Part model, mm, in its own coordinate system. A direction names the side the tool comes from. Give positions to 0.01 mm unless a question says otherwise; leave off trailing zeros. Write each loop counter-clockwise with the first axis right and the second up, starting at its lowest first coordinate (ties: lowest second). Pieces come first, ordered by that corner, then holes. Notation, with made-up numbers: M 85,8.25 L 99,8.25 A9 cw 99,20.25 Z; hole C 66.5,8 d3. An arc over 180 degrees is marked long. Use a Markdown table: item, result. Add a question column.
from build123d import *

# Parameters (mm, degrees)
SKETCH1_W            = 33
SKETCH1_H            = 29
BOSS_EXTRUDE1_DEPTH  = 2
SKETCH2_W            = 33
SKETCH2_H            = 29
SKETCH2_W_2          = 29
SKETCH2_H_2          = 25
BOSS_EXTRUDE2_DEPTH  = 10.5
SKETCH4_W            = 7.5
SKETCH4_H            = 6
CUT_EXTRUDE1_DEPTH   = 2
FILLET1_R            = 2
SKETCH5_W            = 8
SKETCH5_H            = 1
CUT_EXTRUDE2_DEPTH   = 31
FILLET2_R            = 0.5
FILLET2_OF_MIRROR1_R = 0.5


with BuildPart() as part:
    # Sketch1 → Boss-Extrude1 (new body)
    with BuildSketch(Plane(origin=(0, 0, 0), x_dir=(1, 0, 0), z_dir=(0, 1, 0))):
        Rectangle(SKETCH1_W, SKETCH1_H)
    extrude(amount=BOSS_EXTRUDE1_DEPTH)

    # Sketch2 → Boss-Extrude2 (add)
    with BuildSketch(Plane(origin=(0, 2, 0), x_dir=(1, 0, 0), z_dir=(0, 1, 0))):
        Rectangle(SKETCH2_W, SKETCH2_H)
        Rectangle(SKETCH2_W_2, SKETCH2_H_2, mode=Mode.SUBTRACT)
    extrude(amount=BOSS_EXTRUDE2_DEPTH)

    # Sketch4 → Cut-Extrude1 (cut)
    with BuildSketch(Plane(origin=(0, 2, 0), x_dir=(1, 0, 0), z_dir=(0, 1, 0))):
        with Locations((0.05, 4.5)):
            Rectangle(SKETCH4_W, SKETCH4_H)
    extrude(amount=-CUT_EXTRUDE1_DEPTH, mode=Mode.SUBTRACT)

    # Fillet1
    fillet1_edges = [part.edges().sort_by_distance(p)[0] for p in [
        (14.5, 7.25, -12.5),
        (-14.5, 7.25, -12.5),
        (-14.5, 7.25, 12.5),
        (14.5, 7.25, 12.5),
        (16.5, 6.25, 14.5),
        (-16.5, 6.25, 14.5),
        (-16.5, 6.25, -14.5),
        (16.5, 6.25, -14.5),
    ]]
    fillet(fillet1_edges, radius=FILLET1_R)

    # Sketch5 → Cut-Extrude2 (cut)
    with BuildSketch(Plane(origin=(16.5, 0, 0), x_dir=(0, 0, -1), z_dir=(1, 0, 0))):
        with Locations((0, 12)):
            Rectangle(SKETCH5_W, SKETCH5_H)
    cut_extrude2 = extrude(amount=-CUT_EXTRUDE2_DEPTH, mode=Mode.SUBTRACT)

    # Fillet2
    fillet2_edges = [part.edges().sort_by_distance(p)[0] for p in [
        (15.5, 11.5, 4),
        (15.5, 11.5, -4),
    ]]
    fillet(fillet2_edges, radius=FILLET2_R)

    # Mirror1: Cut-Extrude2 across plane
    add(cut_extrude2.mirror(Plane(origin=(0, 0, 0), x_dir=(0, 0, 1), z_dir=(1, 0, 0))), mode=Mode.SUBTRACT)

    # Fillet2 of Mirror1
    fillet2_of_mirror1_edges = [part.edges().sort_by_distance(p)[0] for p in [
        (-15.5, 11.5, 4),
        (-15.5, 11.5, -4),
    ]]
    fillet(fillet2_of_mirror1_edges, radius=FILLET2_OF_MIRROR1_R)


solid = part.part
1. Cut at A-A (x = -1.5). Write the cut outline in (y, z), then the cut area to 3 significant figures.
2. Cut at C-C (y = 3.5). Write the cut outline in (x, z).
3. Tool access for faces 1 (the flat face through (0, 7, 12.5)), 2 (the flat face through (0, 1, -7.5)), 3 (the flat face through (-16, 11.5, 0)): list every direction of +Z, -Z, +X, -X, +Y, -Y with a clear straight run to the whole face (end or side of a thin tool).
4. Drill centre lines: probe 1 along X at (y, z) = (4.75, -9.25); probe 2 along Z at (x, y) = (3, 7); probe 3 along X at (y, z) = (1.5, -2). Where is each one in solid material? Low to high. Write a range as [from, to].
5. Flat gauge pins, fed straight in: pin 1 (1 mm diameter, centred on x = 15.5, z = 1, fed in from +Y); pin 2 (3 mm diameter, centred on x = -10, z = 0, fed in from +Y). Where does each tip first touch, or does it go through?
6. Cut at B-B (z = 8.5). Write the cut outline in (x, y).
7. Cut at D-D (z = -6.25). Write the cut outline in (x, y).
A:
| question | item | result |
|---|---|---|
| 1 | outline | M 0,-14.5 L 12.5,-14.5 L 12.5,-12.5 L 2,-12.5 L 2,-7.5 L 0,-7.5 Z; M 0,-1.5 L 2,-1.5 L 2,12.5 L 12.5,12.5 L 12.5,14.5 L 0,14.5 Z |
| 1 | area | 88.0 mm² |
| 2 | outline | M -16.5,-12.5 A2 ccw -14.5,-14.5 L 14.5,-14.5 A2 ccw 16.5,-12.5 L 16.5,12.5 A2 ccw 14.5,14.5 L -14.5,14.5 A2 ccw -16.5,12.5 Z; hole M -14.5,-10.5 A2 ccw -12.5,-12.5 L 12.5,-12.5 A2 ccw 14.5,-10.5 L 14.5,10.5 A2 ccw 12.5,12.5 L -12.5,12.5 A2 ccw -14.5,10.5 Z |
| 3 | face 1 | +Y |
| 3 | face 2 | +Y, -Y |
| 3 | face 3 | +X, -X, +Y |
| 4 | probe 1 | x = [-16.5, -14.5], [14.5, 16.5] |
| 4 | probe 2 | z = [-14.5, -12.5], [12.5, 14.5] |
| 4 | probe 3 | x = [-16.5, -3.7], [3.8, 16.5] |
| 5 | pin 1 | stops at y = 11.5 |
| 5 | pin 2 | stops at y = 2 |
| 6 | outline | M -16.5,0 L 16.5,0 L 16.5,12.5 L 14.5,12.5 L 14.5,2 L -14.5,2 L -14.5,12.5 L -16.5,12.5 Z |
| 7 | outline | M -16.5,0 L -3.7,0 L -3.7,2 L -14.5,2 L -14.5,12.5 L -16.5,12.5 Z; M 3.8,0 L 16.5,0 L 16.5,12.5 L 14.5,12.5 L 14.5,2 L 3.8,2 Z |
